Print and shaded views of the part. All mm, measured from the part's lowest x, y and z. Round coordinates to 2 decimals unless told otherwise and drop trailing zeros. Write each loop counter-clockwise with the first axis right and the second up, starting at its lowest first coordinate (ties: lowest second). Pieces come first, ordered by that corner, then holes. Notation, with made-up numbers: (3.25, 5.25) - (8.25, 5.25) arc R28 ccw to (8.25, 26.25) - close; hole circle Ø10 at (3.25, 53). An arc over 180 degrees is marked (long way). Put each result on its own line as item: value. Start each with the question number.
Item 1: Cut at A-A (y = 6.25). Give the cut face in (x, z), and give its area (3 significant figures).
Item 2: Pin check, flat tips, straight feed: pin 1 Ø1 at (x, z) = (18, 2) entering from -Y; pin 2 Ø1 at (y, z) = (5, 1.5) entering from +X; pin 3 Ø1 at (x, z) = (24, 0.5) entering from +Y. Stop position of each tip, or through.
Item 3: Cut at D-D (z = 2). Give the cut face in (x, y), and give its area (3 significant figures).
Item 4: Cut at C-C (x = 19.5). Give the cut face in (y, z), and give its area (3 significant figures).
Item 5: Mould opens along Y. For the marked faces 1 and 2 say: released by +Y, released by -Y, zero draft, split by the parting line, or undercut.
Item 6: Cut at B-B (x = 14.5). Give the cut face in (y, z).
Item 7: Drill centre lines: line 1 (X direction, y = 10, z = 1.5); line 2 (X direction, y = 11, z = 1); line 3 (X direction, y = 17.75, z = 1.9). Where is each one in solid material? Low to high. Write a range as from..to.
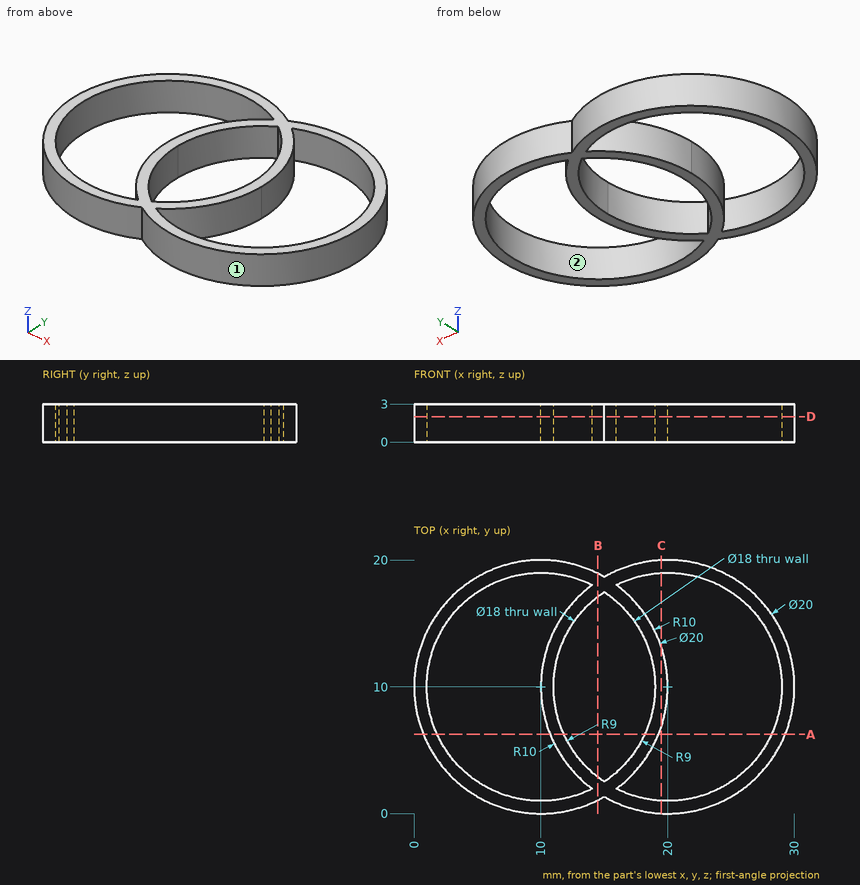
Output values:
1. outline: (0.73, 0) - (1.82, 0) - (1.82, 3) - (0.73, 3) - close; (10.73, 0) - (11.82, 0) - (11.82, 3) - (10.73, 3) - close; (18.18, 0) - (19.27, 0) - (19.27, 3) - (18.18, 3) - close; (28.18, 0) - (29.27, 0) - (29.27, 3) - (28.18, 3) - close
1. area: 13.1 mm2
2. pin 1: y = 0.11
2. pin 2: x = 28.93
2. pin 3: y = 19.37
3. outline: (15, 1.34) arc R10 ccw (long way) to (15, 18.66) arc R10 ccw (long way) to start; hole (10, 10) arc R10 cw to (14.05, 18.04) arc R9 ccw (long way) to (14.05, 1.96) arc R10 cw to start; hole (11, 10) arc R9 ccw to (15, 2.52) arc R9 ccw to (19, 10) arc R9 ccw to (15, 17.48) arc R9 ccw to start; hole (15.95, 1.96) arc R9 ccw (long way) to (15.95, 18.04) arc R10 cw to (20, 10) arc R10 cw to start
3. area: 117 mm2
4. outline: (0.01, 0) - (1.01, 0) - (1.01, 3) - (0.01, 3) - close; (6.88, 0) - (13.12, 0) - (13.12, 3) - (6.88, 3) - close; (18.99, 0) - (19.99, 0) - (19.99, 3) - (18.99, 3) - close
4. area: 24.7 mm2
5. face 1: split by the parting line
5. face 2: undercut
6. outline: (1.07, 0) - (2.88, 0) - (2.88, 3) - (1.07, 3) - close; (17.12, 0) - (18.93, 0) - (18.93, 3) - (17.12, 3) - close
7. line 1: 0..1, 10..11, 19..20, 29..30
7. line 2: 0.05..1.06, 10.05..11.06, 18.94..19.95, 28.94..29.95
7. line 3: 3.68..5.42, 13.68..16.32, 24.58..26.32
